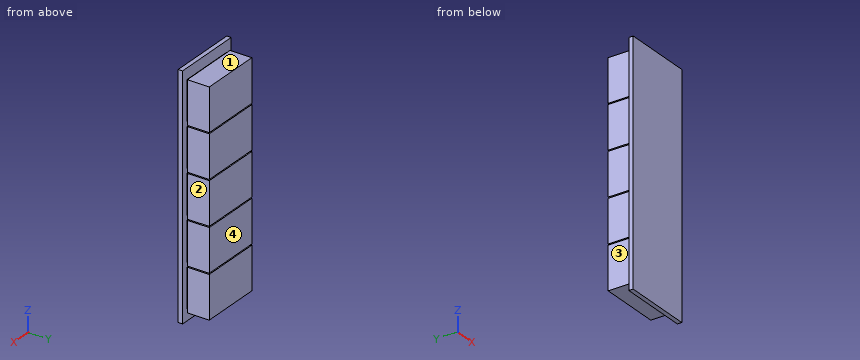
```python
from build123d import *

# Parameters (mm, degrees)
SKETCH1_W           = 80
SKETCH1_H           = 270
BOSS_EXTRUDE1_DEPTH = 5
SKETCH2_W           = 65
SKETCH2_H           = 45
BOSS_EXTRUDE3_DEPTH = 2
LPATTERN1_COUNT     = 5
LPATTERN1_PITCH     = 50
SKETCH3_W           = 70
SKETCH3_H           = 48.748964222
BOSS_EXTRUDE8_DEPTH = 25
LPATTERN5_COUNT     = 5
LPATTERN5_PITCH     = 50


with BuildPart() as part:
    # Sketch1 → Boss-Extrude1 (new body)
    with BuildSketch(Plane(origin=(0, 0, 0), x_dir=(1, 0, 0), z_dir=(0, 1, 0))):
        Rectangle(SKETCH1_W, SKETCH1_H)
    extrude(amount=BOSS_EXTRUDE1_DEPTH)

    # Sketch2 → Boss-Extrude3 (add)
    with BuildSketch(Plane(origin=(0, 5, 0), x_dir=(1, 0, 0), z_dir=(0, 1, 0))):
        with Locations((0, -100)):
            Rectangle(SKETCH2_W, SKETCH2_H)
    boss_extrude3 = extrude(amount=BOSS_EXTRUDE3_DEPTH)

    # LPattern1: Boss-Extrude3 ×5
    with Locations(*[(0, 0, -i * LPATTERN1_PITCH) for i in range(1, LPATTERN1_COUNT)]):
        add(boss_extrude3)

    # Sketch3 → Boss-Extrude8 (add)
    with BuildSketch(Plane(origin=(0, 7, 0), x_dir=(1, 0, 0), z_dir=(0, 1, 0))):
        with Locations((0, -99.635002086)):
            Rectangle(SKETCH3_W, SKETCH3_H)
    boss_extrude8 = extrude(amount=BOSS_EXTRUDE8_DEPTH)

    # LPattern5: Boss-Extrude8 ×5
    with Locations(*[(0, 0, -i * LPATTERN5_PITCH) for i in range(1, LPATTERN5_COUNT)]):
        add(boss_extrude8)


solid = part.part
```
The listing builds one solid part. Answer for the finished solid, in the listing's coordinates (mm). Face numbers are marked on the shaded views. A direction names the side the tool comes from. Give positions to 0.01 mm unless a question says otherwise; leave off trailing zeros. Write each loop counter-clockwise with the first axis right and the second up, starting at its lowest first coordinate (ties: lowest second). Pieces come first, ordered by that corner, then holes. Notation, with made-up numbers: (-30.5, 52.5) -> (-15.5, 52.5) arc R18 ccw to (-15.5, 68.5) -> close; hole circle Ø11 at (75.25, 25.5). An arc over 180 degrees is marked (long way). Write item = value, one per line. Start each with the question number.
1) Which of the six approach directions +Z, -Z, +X, -X, +Y, -Y give full straight-line access (tool end or side, diameter ignored) to the marked faces 1, 2, 3 and 4?
2) Each of these flat-tipped pins is pushed along its axis until it touches: pin 1 (6 mm diameter, centred on y = 11.5, z = 98.5, fed in from -X); pin 2 (4 mm diameter, centred on y = 7.5, z = -96.5, fed in from +X); pin 3 (7.5 mm diameter, centred on x = -16, y = 20.5, fed in from +Z). Where does it stop, or does it pass through?
3) Straight lines are drawn through the part: line 1 along Z through (x, y) = (13, 30); line 2 along Y through (x, z) = (27.5, 73); line 3 along Y through (x, z) = (6, 25). For each, find the intervals that lie inside material, in ascending order.
4) The part is cut by section B-B, the plane z = -2.5. Determine the outline of the cut face in (x, y).
5) The part is cut by section A-A, the plane y = 16.5. Determine the outline of the cut face in (x, z), and give its area (3 significant figures).
Solutions:
q1.face_1 = +Z, +X, -X, +Y
q1.face_2 = +Z, -Z, +X, +Y
q1.face_3 = +Z, -Z, -X, +Y
q1.face_4 = +Z, -Z, +X, -X, +Y
q2.pin_1 = -35
q2.pin_2 = 35
q2.pin_3 = 124.01
q3.line_1 = -124.74 to -75.99, -74.74 to -25.99, -24.74 to 24.01, 25.26 to 74.01, 75.26 to 124.01
q3.line_2 = 0 to 5, 7 to 32
q3.line_3 = 0 to 5
q4.outline = (-40, 0) -> (40, 0) -> (40, 5) -> (32.5, 5) -> (32.5, 7) -> (35, 7) -> (35, 32) -> (-35, 32) -> (-35, 7) -> (-32.5, 7) -> (-32.5, 5) -> (-40, 5) -> close
q5.outline = (-35, -124.74) -> (35, -124.74) -> (35, -75.99) -> (-35, -75.99) -> close; (-35, -74.74) -> (35, -74.74) -> (35, -25.99) -> (-35, -25.99) -> close; (-35, -24.74) -> (35, -24.74) -> (35, 24.01) -> (-35, 24.01) -> close; (-35, 25.26) -> (35, 25.26) -> (35, 74.01) -> (-35, 74.01) -> close; (-35, 75.26) -> (35, 75.26) -> (35, 124.01) -> (-35, 124.01) -> close
q5.area = 17,100 mm²
